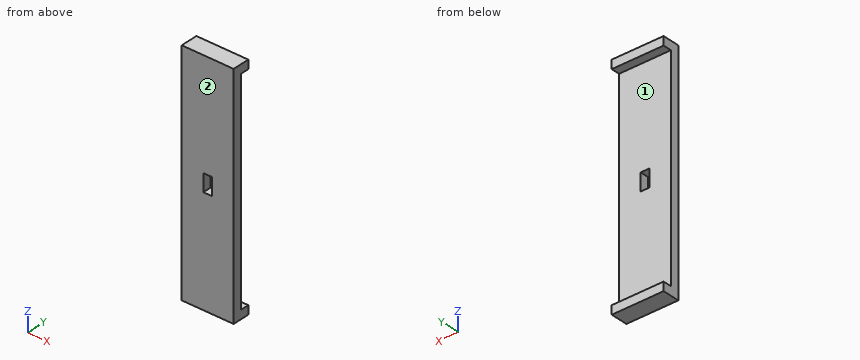
```python
from build123d import *

# Parameters (mm, degrees)
SKETCH1_W           = 18
SKETCH1_H           = 80
SKETCH1_W_2         = 3
SKETCH1_H_2         = 6
BOSS_EXTRUDE1_DEPTH = 3
SKETCH2_W           = 18
SKETCH2_H           = 3
BOSS_EXTRUDE2_DEPTH = 3


with BuildPart() as part:
    # Sketch1 → Boss-Extrude1 (new body)
    with BuildSketch(Plane(origin=(0, 0, 0), x_dir=(1, 0, 0), z_dir=(0, 1, 0))):
        Rectangle(SKETCH1_W, SKETCH1_H)
        Rectangle(SKETCH1_W_2, SKETCH1_H_2, mode=Mode.SUBTRACT)
    extrude(amount=BOSS_EXTRUDE1_DEPTH)

    # Sketch2 → Boss-Extrude2 (add)
    with BuildSketch(Plane(origin=(0, 3, 0), x_dir=(1, 0, 0), z_dir=(0, 1, 0))):
        with Locations((0, -38.5)):
            Rectangle(SKETCH2_W, SKETCH2_H)
        with Locations((0, 38.5)):
            Rectangle(SKETCH2_W, SKETCH2_H)
    extrude(amount=BOSS_EXTRUDE2_DEPTH)


solid = part.part
```
Model file for the job. Use its own axes, mm. Face numbers are marked on the shaded views. Coordinates: 2 decimals unless noted, no trailing zeros. Order: outer loops, then holes, each group sorted by start corner. A loop starts at its lowest first (then second) coordinate and runs counter-clockwise, first axis right, second up. Notation, with made-up numbers: (55, -12) -> (96, -12) arc R11 ccw to (96, 7) -> close; hole circle Ø2 at (-30.5, -35.75). An arc over 180 degrees is marked (long way). Answer as a JSON object with one key per item and string values. Group by question number.
1) Flat gauge pin, fed straight in: pin 1 (8 mm diameter, centred on x = -1.5, z = 12, fed in from -Y). Where does the tip first touch, or does it go through?
2) Drill centre lines: L1, parallel to Z at x = 0, y = 2.6; L2, parallel to Z at x = -3.5, y = 4.5; L3, parallel to X at y = 2.4, z = 2. Where is each one in solid material? Low to high.
3) Cut at C-C, the plane x = -7.25. Write the cut outline in (y, z).
4) Cut at D-D, the plane z = 14. Write the cut outline in (x, y).
5) Pull direction Z, two halves, no side cores. Call the marked faces 1 and 2: +Z half, -Z half, draft (parallel to the pull), parting line (faces both ways), or undercut.
6) Cut at B-B, the plane x = 0.5. Write the cut outline in (y, z).
7) Cut at A-A, the plane y = 4.6. Write the cut outline in (x, z), then the cut area to 3 significant figures.
Check values:
{
 "1": {"pin 1": "stops at y = 0"},
 "2": {"L1": "z = -40 to -3, 3 to 40", "L2": "z = -40 to -37, 37 to 40", "L3": "x = -9 to -1.5, 1.5 to 9"},
 "3": {"outline": "(0, -40) -> (6, -40) -> (6, -37) -> (3, -37) -> (3, 37) -> (6, 37) -> (6, 40) -> (0, 40) -> close"},
 "4": {"outline": "(-9, 0) -> (9, 0) -> (9, 3) -> (-9, 3) -> close"},
 "5": {"face 1": "undercut", "face 2": "draft"},
 "6": {"outline": "(0, -40) -> (6, -40) -> (6, -37) -> (3, -37) -> (3, -3) -> (0, -3) -> close; (0, 3) -> (3, 3) -> (3, 37) -> (6, 37) -> (6, 40) -> (0, 40) -> close"},
 "7": {"outline": "(-9, -40) -> (9, -40) -> (9, -37) -> (-9, -37) -> close; (-9, 37) -> (9, 37) -> (9, 40) -> (-9, 40) -> close", "area": "108 mm²"}
}
